```python
from build123d import *

# Parameters (mm, degrees)
F1_DEPTH = 12.7
F3_DEPTH = 25.4
F5_DEPTH = 25.4
F7_DEPTH = 25.4
F9_DEPTH = 25.4


with BuildPart() as f1:
    # F0 (on Top) → F1 (new body)
    with BuildSketch(Plane.XY):
        with BuildLine():
            Line((-2.004466, 3.509337), (2.036942, 3.490587))
            Line((2.036942, 3.490587), (4.041408, -0.01875))
            Line((4.041408, -0.01875), (4.041408, 0.564419))
            Line((4.041408, 0.564419), (4.530986, 0.564419))
            ThreePointArc((4.530986, 0.564419), (3.029542, 3.41618), (0.01875, 4.565967))
            Line((0.01875, 4.565967), (0.01875, 4.041408))
            Line((0.01875, 4.041408), (-0.564419, 4.041408))
            Line((-0.564419, 4.041408), (-0.564419, 4.530986))
            ThreePointArc((-0.564419, 4.530986), (-3.41618, 3.029542), (-4.565967, 0.01875))
            Line((-4.565967, 0.01875), (-4.041408, 0.01875))
            Line((-4.041408, 0.01875), (-2.004466, 3.509337))
        make_face()
        with BuildLine():
            ThreePointArc((4.566005, 0), (4.565996, -0.009375), (4.565967, -0.01875))
            Line((4.565967, -0.01875), (6.073408, -0.01875))
            Line((6.073408, -0.01875), (6.073408, 0.564419))
            Line((6.073408, 0.564419), (4.530986, 0.564419))
            ThreePointArc((4.530986, 0.564419), (4.557242, 0.282752), (4.566005, 0))
        make_face()
        with BuildLine():
            Line((4.041408, 0.564419), (4.041408, -0.01875))
            Line((4.041408, -0.01875), (4.565967, -0.01875))
            ThreePointArc((4.565967, -0.01875), (4.565996, -0.009375), (4.566005, 0))
            ThreePointArc((4.566005, 0), (4.557242, 0.282752), (4.530986, 0.564419))
            Line((4.530986, 0.564419), (4.041408, 0.564419))
        make_face()
        with BuildLine():
            ThreePointArc((-0.564419, 4.530986), (-0.273394, 4.557813), (0.01875, 4.565967))
            Line((0.01875, 4.565967), (0.01875, 6.073408))
            Line((0.01875, 6.073408), (-0.564419, 6.073408))
            Line((-0.564419, 6.073408), (-0.564419, 4.530986))
        make_face()
        with BuildLine():
            Line((0.01875, 4.041408), (0.01875, 4.565967))
            ThreePointArc((0.01875, 4.565967), (-0.273394, 4.557813), (-0.564419, 4.530986))
            Line((-0.564419, 4.530986), (-0.564419, 4.041408))
            Line((-0.564419, 4.041408), (0.01875, 4.041408))
        make_face()
        with BuildLine():
            ThreePointArc((-4.530986, -0.564419), (-4.557813, -0.273394), (-4.565967, 0.01875))
            Line((-4.565967, 0.01875), (-6.073408, 0.01875))
            Line((-6.073408, 0.01875), (-6.073408, -0.564419))
            Line((-6.073408, -0.564419), (-4.530986, -0.564419))
        make_face()
        with BuildLine():
            Line((-4.041408, -0.564419), (-4.041408, 0.01875))
            Line((-4.041408, 0.01875), (-4.565967, 0.01875))
            ThreePointArc((-4.565967, 0.01875), (-4.557813, -0.273394), (-4.530986, -0.564419))
            Line((-4.530986, -0.564419), (-4.041408, -0.564419))
        make_face()
        with BuildLine():
            Line((4.565967, -0.01875), (4.041408, -0.01875))
            Line((4.041408, -0.01875), (2.004466, -3.509337))
            Line((2.004466, -3.509337), (-2.036942, -3.490587))
            Line((-2.036942, -3.490587), (-4.041408, 0.01875))
            Line((-4.041408, 0.01875), (-4.041408, -0.564419))
            Line((-4.041408, -0.564419), (-4.530986, -0.564419))
            ThreePointArc((-4.530986, -0.564419), (-3.029542, -3.41618), (-0.01875, -4.565967))
            Line((-0.01875, -4.565967), (-0.01875, -4.041408))
            Line((-0.01875, -4.041408), (0.564419, -4.041408))
            Line((0.564419, -4.041408), (0.564419, -4.530986))
            ThreePointArc((0.564419, -4.530986), (3.41618, -3.029542), (4.565967, -0.01875))
        make_face()
        with BuildLine():
            ThreePointArc((-0.01875, -4.565967), (0.273394, -4.557813), (0.564419, -4.530986))
            Line((0.564419, -4.530986), (0.564419, -4.041408))
            Line((0.564419, -4.041408), (-0.01875, -4.041408))
            Line((-0.01875, -4.041408), (-0.01875, -4.565967))
        make_face()
        with BuildLine():
            Line((0.564419, -6.073408), (0.564419, -4.530986))
            ThreePointArc((0.564419, -4.530986), (0.273394, -4.557813), (-0.01875, -4.565967))
            Line((-0.01875, -4.565967), (-0.01875, -6.073408))
            Line((-0.01875, -6.073408), (0.564419, -6.073408))
        make_face()
    extrude(amount=F1_DEPTH)

    # F2 (on face) → F3 (cut)
    with BuildSketch(Plane.XZ.offset(0.01875)):
        Polygon((6.073408, 0), (6.073408, 12.7), (4.565967, 0), align=None)
    extrude(amount=-F3_DEPTH, mode=Mode.SUBTRACT)

    # F4 (on face) → F5 (cut)
    with BuildSketch(Plane(origin=(-0.01875, 0, 0), x_dir=(0, -1, 0), z_dir=(-1, 0, 0))):
        Polygon((6.073408, 0), (6.073408, 12.7), (4.565967, 0), align=None)
    extrude(amount=-F5_DEPTH, mode=Mode.SUBTRACT)

    # F6 (on face) → F7 (cut)
    with BuildSketch(Plane.YZ.offset(0.01875)):
        Polygon((6.073408, 0), (6.073408, 12.7), (4.565967, 0), align=None)
    extrude(amount=-F7_DEPTH, mode=Mode.SUBTRACT)

    # F8 (on face) → F9 (cut)
    with BuildSketch(Plane(origin=(0, 0.01875, 0), x_dir=(-1, 0, 0), z_dir=(0, 1, 0))):
        Polygon((6.073408, 0), (6.073408, 12.7), (4.565967, 0), align=None)
    extrude(amount=-F9_DEPTH, mode=Mode.SUBTRACT)


solid = f1.part
```
Model file for the job. Use its own axes, mm. A direction names the side the tool comes from. Round coordinates to 2 decimals unless told otherwise and drop trailing zeros. Write each loop counter-clockwise with the first axis right and the second up, starting at its lowest first coordinate (ties: lowest second). Pieces come first, ordered by that corner, then holes. Notation, with made-up numbers: (29, 48) - (39, 48) arc R20 cw to (39, 75) - close; hole circle Ø3 at (10, 38). An arc over 180 degrees is marked (long way). Use CSV: the item, a comma, the result in double quotes. Start each with the question number.
Item 1: Tool access for faces 1 (the face through (-0.019, -5, 9)), 2 (the face through (5, -0.019, 9)), 3 (the face through (-3.037, 1.74, 6.261)), 4 (the face through (5, 0.564, 8)): list every direction of +Z, -Z, +X, -X, +Y, -Y with a clear straight run to the whole face (end or side of a thin tool).
Item 2: Drill centre lines: L1, parallel to Y at x = 5.5, z = 8.5; L2, parallel to Y at x = 3, z = 5.75; L3, parallel to Y at x = -1, z = 4.75. Where is each one in solid material? Low to high. Write a range as [from, to].
Item 3: Band-saw the part on B-B (x = 1). Write the cut outline in (y, z), and give its area (3 significant figures).
Item 4: Band-saw the part on A-A (y = -1). Write the cut outline in (x, z), and give its area (3 significant figures).
Item 5: Pin check, flat tips, straight feed: P1, Ø6, axis at y = -4, z = 5.5, coming from the +X side; P2, Ø1.5, axis at y = 0, z = 7, coming from the -X side; P3, Ø0.5, axis at y = 5.5, z = 6.5, coming from the -X side. Stop position of each tip, or through.
Item 6: Band-saw the part on D-D (z = 9.25). Write the cut outline in (x, y).
Item 7: Two-plate mould, pull along X, no slides. Class faces 5 (the face through (0.019, 5, 9)), 6 (the face through (-5, -0.564, 8)), 7 (the face through (-3.025, -1.76, 6.261)), 8 (the face through (-0.564, 5, 8)): released by +X, released by -X, zero draft, split by the parting line, or undercut.
Item 8: Band-saw the part on C-C (z = 6.25). Write the cut outline in (x, y), and give its area (3 significant figures).
Checked values:
1,face 1,"+Z, -Z, -X, -Y"
1,face 2,"+Z, -Z, +X, -Y"
1,face 3,"+Z, -Z"
1,face 4,"+Z, -Z, +X, +Y"
2,L1,"y = [-0.02, 0.56]"
2,L2,"y = [-3.44, -1.8], [1.8, 3.44]"
2,L3,"y = [-4.46, -3.5], [3.5, 4.46]"
3,outline,"(-4.46, 0) - (-3.5, 0) - (-3.5, 12.7) - (-4.46, 12.7) - close; (3.5, 0) - (4.46, 0) - (4.46, 12.7) - (3.5, 12.7) - close"
3,area,"24.3 mm²"
4,outline,"(-4.46, 0) - (-3.46, 0) - (-3.46, 12.7) - (-4.46, 12.7) - close; (3.47, 0) - (4.46, 0) - (4.46, 12.7) - (3.47, 12.7) - close"
4,area,"25.2 mm²"
5,P1,"stops at x = 4.46"
5,P2,"stops at x = -5.49"
5,P3,"stops at x = -0.56"
6,outline,"(-5.66, -0.56) - (-4.53, -0.56) arc R4.57 ccw to (-0.02, -4.57) - (-0.02, -5.66) - (0.56, -5.66) - (0.56, -4.53) arc R4.57 ccw to (4.57, -0.02) - (5.66, -0.02) - (5.66, 0.56) - (4.53, 0.56) arc R4.57 ccw to (0.02, 4.57) - (0.02, 5.66) - (-0.56, 5.66) - (-0.56, 4.53) arc R4.57 ccw to (-4.57, 0.02) - (-5.66, 0.02) - close; hole (-4.04, 0.02) - (-2.04, -3.49) - (2, -3.51) - (4.04, -0.02) - (2.04, 3.49) - (-2, 3.51) - close"
7,face 5,"released by +X"
7,face 6,"zero draft"
7,face 7,"undercut"
7,face 8,"released by -X"
8,outline,"(-5.31, -0.56) - (-4.53, -0.56) arc R4.57 ccw to (-0.02, -4.57) - (-0.02, -5.31) - (0.56, -5.31) - (0.56, -4.53) arc R4.57 ccw to (4.57, -0.02) - (5.31, -0.02) - (5.31, 0.56) - (4.53, 0.56) arc R4.57 ccw to (0.02, 4.57) - (0.02, 5.31) - (-0.56, 5.31) - (-0.56, 4.53) arc R4.57 ccw to (-4.57, 0.02) - (-5.31, 0.02) - close; hole (-4.04, 0.02) - (-2.04, -3.49) - (2, -3.51) - (4.04, -0.02) - (2.04, 3.49) - (-2, 3.51) - close"
8,area,"24.8 mm²"
